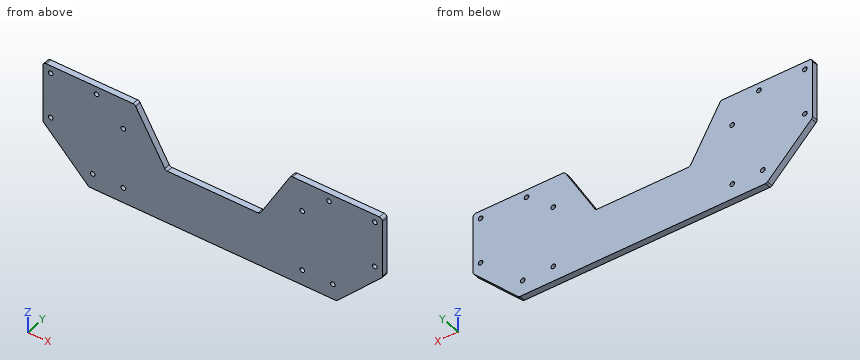
from build123d import *

# Parameters (mm, degrees)
EXTRUDE_1_DEPTH     = 4
SKETCH_2_R          = 1.5
CUT_EXTRUDE_1_DEPTH = 10
FILLET_2_R          = 2


with BuildPart() as part:
    # 草图1 → 凸台-拉伸1 (new body)
    with BuildSketch(Plane(origin=(0, 0, 0), x_dir=(1, 0, 0), z_dir=(0, 1, 0))):
        Polygon((-80.207259422, 5), (-80.207259422, -35), (-20.207259422, -35), (0, 0), (61.585481157, 0), (81.792740578, -35), (141.792740578, -35), (141.792740578, 5), (111.792740578, 35), (-50.207259422, 35), align=None)
    extrude(amount=EXTRUDE_1_DEPTH)

    # 草图2 → 切除-拉伸1 (cut)
    with BuildSketch(Plane(origin=(0, 4, 0), x_dir=(1, 0, 0), z_dir=(0, 1, 0))):
        with Locations(Location((-27.707259422, -15, 0), (0, 0, 270))):
            Circle(SKETCH_2_R)
        with Locations(Location((-27.707259422, 25, 0), (0, 0, 270))):
            Circle(SKETCH_2_R)
        with Locations(Location((-75.207259422, -30, 0), (0, 0, 270))):
            Circle(SKETCH_2_R)
        with Locations(Location((-45.207259422, -30, 0), (0, 0, 270))):
            Circle(SKETCH_2_R)
        with Locations(Location((-75.207259422, 0, 0), (0, 0, 270))):
            Circle(SKETCH_2_R)
        with Locations(Location((-47.707259422, 25, 0), (0, 0, 270))):
            Circle(SKETCH_2_R)
        with Locations(Location((109.292740578, 25, 0), (0, 0, 90))):
            Circle(SKETCH_2_R)
        with Locations(Location((136.792740578, 0, 0), (0, 0, 90))):
            Circle(SKETCH_2_R)
        with Locations(Location((106.792740578, -30, 0), (0, 0, 90))):
            Circle(SKETCH_2_R)
        with Locations(Location((136.792740578, -30, 0), (0, 0, 90))):
            Circle(SKETCH_2_R)
        with Locations(Location((89.292740578, 25, 0), (0, 0, 90))):
            Circle(SKETCH_2_R)
        with Locations(Location((89.292740578, -15, 0), (0, 0, 90))):
            Circle(SKETCH_2_R)
    extrude(amount=-CUT_EXTRUDE_1_DEPTH, mode=Mode.SUBTRACT)

    # 圆角2
    fillet_2_edges = [part.edges().sort_by_distance(p)[0] for p in [
        (-50.207259422, 2, -35),
        (111.792740578, 2, -35),
        (141.792740578, 2, -5),
        (141.792740578, 2, 35),
        (81.792740578, 2, 35),
        (61.585481157, 2, 0),
        (0, 2, 0),
        (-20.207259422, 2, 35),
        (-80.207259422, 2, 35),
        (-80.207259422, 2, -5),
    ]]
    fillet(fillet_2_edges, radius=FILLET_2_R)


solid = part.part
Here's how the part is built. I have some questions about the finished solid (model axes, mm). Coordinates: 2 decimals unless noted, no trailing zeros. Order: outer loops, then holes, each group sorted by start corner. A loop starts at its lowest first (then second) coordinate and runs counter-clockwise, first axis right, second up. Notation, with made-up numbers: (12, -35) - (62, -35) arc R23 ccw to (62, -5) - close; hole circle Ø11 at (4, 77). An arc over 180 degrees is marked (long way). Use CSV: the item, a comma, the result in double quotes. Start each with the question number.
1. Please list where these lines run through material, in increasing order: line 1 (X direction, y = 1, z = 15); line 2 (X direction, y = 2.6, z = 30); line 3 (X direction, y = 3.85, z = 31). Write a range as from..to.
2. Suppose I cut it at A-A on y = 1.05. Give the number of separate pieces and of enclosed holes in the cut face, then the cut area to 3 significant figures.
3. I'm going to push flat-ended pins straight in: pin 1 (3 mm diameter, centred on x = -54.5, z = 19, fed in from -Y); pin 2 (1.2 mm diameter, centred on x = 19.5, y = 2.5, fed in from +Z); pin 3 (2.5 mm diameter, centred on x = -47.71, z = -25, fed in from -Y). Where does each tip first touch, or does it pass through?
4. Suppose I cut it at B-B on x = 26. List the corners of the cut face in (y, z) for me, then the cut area to 3 significant figures.
5. Suppose I cut it at C-C on x = -8. List the corners of the cut face in (y, z) for me, then the cut area to 3 significant figures.
Output:
1,line 1,"x = -80.21..-29.21, -26.21..-8.66, 70.25..87.79, 90.79..141.79"
1,line 2,"x = -80.21..-76.71, -73.71..-46.71, -43.71..-17.32, 78.91..105.29, 108.29..135.29, 138.29..141.79"
1,line 3,"x = -80.21..-76.33, -74.09..-46.33, -44.09..-17.9, 79.48..105.67, 107.91..135.67, 137.91..141.79"
2,separate pieces,"1"
2,enclosed holes,"12"
2,area,"11,700 mm2"
3,pin 1,"stops at y = 0"
3,pin 2,"stops at z = 0"
3,pin 3,"passes through"
4,outline,"(0, -35) - (4, -35) - (4, 0) - (0, 0) - close"
4,area,"140 mm2"
5,outline,"(0, -35) - (4, -35) - (4, 13.86) - (0, 13.86) - close"
5,area,"195 mm2"
